Source: CAD feature listing. Evaluate the final solid. Frame: model axes, mm. Face numbers are marked on the shaded views. A direction names the side the tool comes from. Coordinates: 2 decimals unless noted, no trailing zeros. Order: outer loops, then holes, each group sorted by start corner. A loop starts at its lowest first (then second) coordinate and runs counter-clockwise, first axis right, second up. Notation, with made-up numbers: (-29, 78) -> (-18, 78) arc R23 cw to (-18, 108) -> close; hole circle Ø8 at (46.25, 21). An arc over 180 degrees is marked (long way). Write item = value, one per line. Start each with the question number.
Item 1: Ray query, line 1 along X through (y, z) = (2.55, 0) (3 decimals); line 2 along X through (y, z) = (5.25, 0) (3 decimals); line 3 along Z through (x, y) = (6.35, 6.75) (3 decimals). Return the intervals inside material, ascending. Write a range as [from, to].
Item 2: Section query B-B (x = 9.5). Output: boundary loops of the cut face in (y, z) (3 decimals).
Item 3: Contact query for flat-ended pins moving along their axis: pin 1 (1.7 mm diameter, centred on x = 6, z = 0, fed in from +Y) (3 decimals); pin 2 (1 mm diameter, centred on y = 6.5, z = -0.5, fed in from -X) (3 decimals); pin 3 (2 mm diameter, centred on x = 3, z = -0.5, fed in from -Y). Output: stop coordinate, or through.
Item 4: Set-up query: the marked faces 1 and 2. Return all of +Z, -Z, +X, -X, +Y, -Y with unobstructed straight access to the full face (end or side cutting, diameter ignored); none if empty.
Item 5: Mould query, pull axis X, two halves, no side actions, for the marked faces 3, 4, 5 and 6. Classes: released by +X, released by -X, zero draft, split by the parting line, or undercut.
Item 6: Section query D-D (x = 5.75). Output: boundary loops of the cut face in (y, z) (3 decimals).
Item 7: Section query C-C (z = 3.5). Output: boundary loops of the cut face in (x, y) (3 decimals).
Item 8: Section query A-A (y = 6). Output: boundary loops of the cut face in (x, z) (3 decimals).
```python
from build123d import *

# Parameters (mm, degrees)
SKETCH1_R           = 1.651
BOSS_EXTRUDE1_DEPTH = 3.175
SKETCH2_R           = 4.445
SKETCH2_R_2         = 1.651
BOSS_EXTRUDE2_DEPTH = 7.366


with BuildPart() as part:
    # Sketch1 → Boss-Extrude1 (new body)
    with BuildSketch(Plane(origin=(0, 0, 0), x_dir=(1, 0, 0), z_dir=(0, 1, 0))):
        with BuildLine():
            Line((0, 4.445), (12.7, 4.445))
            ThreePointArc((12.7, 4.445), (17.145, 0), (12.7, -4.445))
            Line((12.7, -4.445), (0, -4.445))
            ThreePointArc((0, -4.445), (-4.445, 0), (0, 4.445))
        make_face()
        with Locations((12.7, 0)):
            Circle(SKETCH1_R, mode=Mode.SUBTRACT)
        Circle(SKETCH1_R, mode=Mode.SUBTRACT)
    extrude(amount=BOSS_EXTRUDE1_DEPTH)

    # Sketch2 → Boss-Extrude2 (add)
    with BuildSketch(Plane(origin=(0, 3.175, 0), x_dir=(1, 0, 0), z_dir=(0, 1, 0))):
        with Locations((6.35, 0)):
            Circle(SKETCH2_R)
        with Locations((6.35, 0)):
            Circle(SKETCH2_R_2, mode=Mode.SUBTRACT)
    extrude(amount=BOSS_EXTRUDE2_DEPTH)


solid = part.part
```
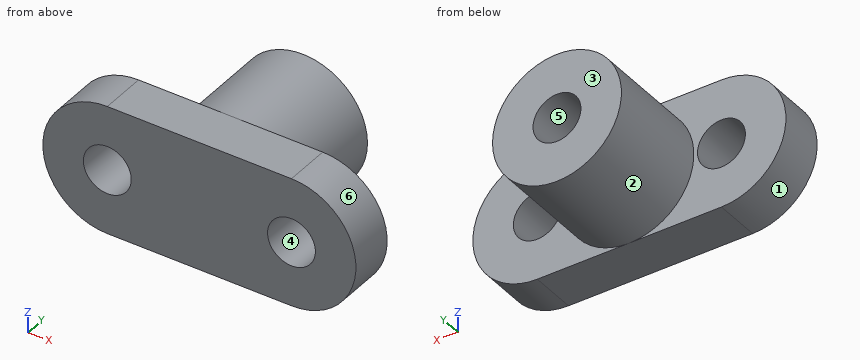
Computed:
q1.line_1 = [-4.445, -1.651], [1.651, 11.049], [14.351, 17.145]
q1.line_2 = [1.905, 4.699], [8.001, 10.795]
q1.line_3 = [-4.445, -1.651], [1.651, 4.445]
q2.outline = (0, -4.445) -> (3.175, -4.445) -> (3.175, -3.136) -> (10.541, -3.136) -> (10.541, 3.136) -> (3.175, 3.136) -> (3.175, 4.445) -> (0, 4.445) -> close
q3.pin_1 = 3.175
q3.pin_2 = 1.905
q3.pin_3 = 0
q4.face_1 = -X, +Y, -Y
q4.face_2 = +Y
q5.face_3 = zero draft
q5.face_4 = undercut
q5.face_5 = undercut
q5.face_6 = released by +X
q6.outline = (0, -4.445) -> (3.175, -4.445) -> (3.175, -4.404) -> (10.541, -4.404) -> (10.541, -1.538) -> (3.175, -1.538) -> (3.175, 1.538) -> (10.541, 1.538) -> (10.541, 4.404) -> (3.175, 4.404) -> (3.175, 4.445) -> (0, 4.445) -> close
q7.outline = (-2.74, 0) -> (15.44, 0) -> (15.44, 3.175) -> (9.09, 3.175) -> (9.09, 10.541) -> (3.61, 10.541) -> (3.61, 3.175) -> (-2.74, 3.175) -> close
q8.outline = circle Ø8.89 at (6.35, 0); hole circle Ø3.302 at (6.35, 0)
